The drawing under review shows one solid part. Ordinate dimensions are in mm from its lowest x, y, z. A direction names the side the tool comes from. Coordinates: 2 decimals unless noted, no trailing zeros. Order: outer loops, then holes, each group sorted by start corner. A loop starts at its lowest first (then second) coordinate and runs counter-clockwise, first axis right, second up. Notation, with made-up numbers: (39, 65) - (98, 65) arc R29 ccw to (98, 100) - close; hole circle Ø10 at (34, -11). An arc over 180 degrees is marked (long way). Write each question's results on one line, items separated by ' | '. Start each with the question number.
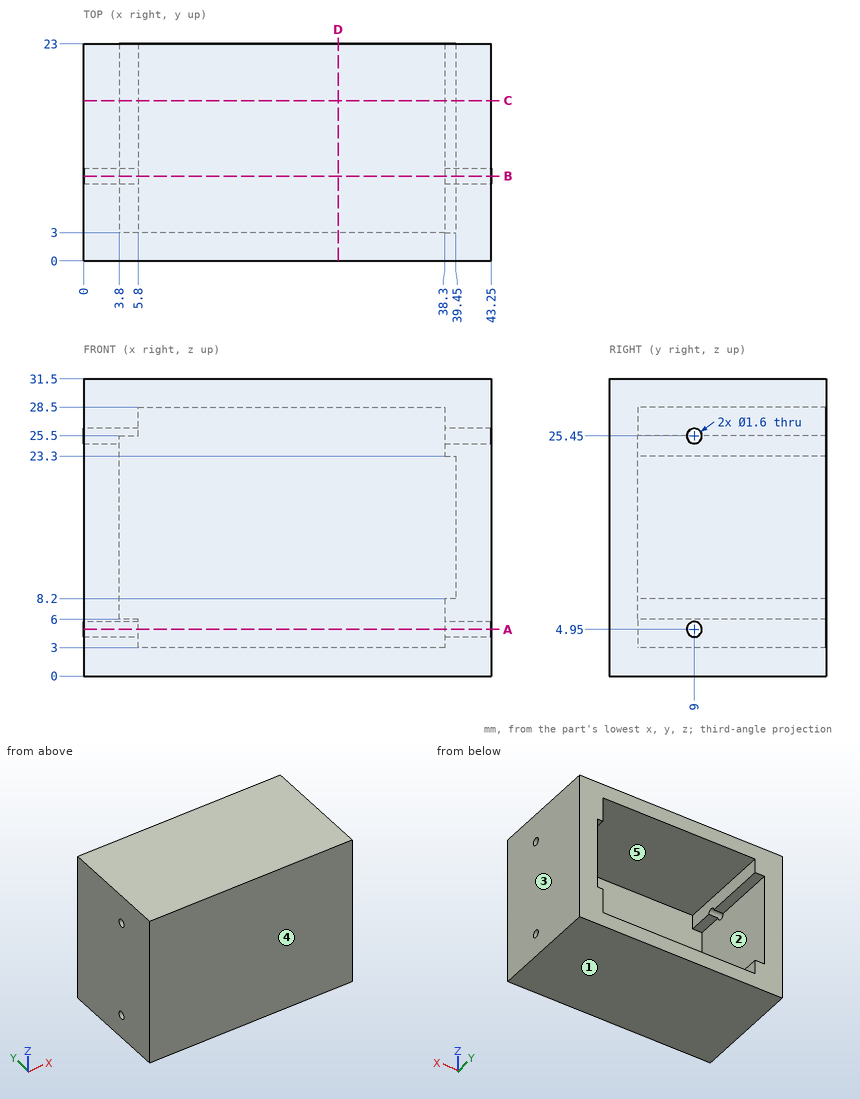
(1) Take a section at C-C (y = 17). State the section outline as (x, z) points, plus the area to 3 significant figures.
(2) To check wall thickness, follow line 1 along Z through (x, y) = (4.2, 9); line 2 along Z through (x, y) = (39.7, 9); line 3 along Y through (x, z) = (2.4, 4.95). State the ranges of each line that lie inside material, in increasing order. Write a range as [from, to].
(3) Take a section at D-D (x = 27). State the section outline as (y, z) points, plus the area to 4 significant figures.
(4) Take a section at B-B (y = 9). State how many separate pieces and enclosed holes the cut face has, plus the area to 3 significant figures.
(5) Mouldability with a two-part tool opening along X and no side actions: class the marked faces 1, 2 and 3 as +X half, -X half, draft (parallel to the pull), parting line (faces both ways), or undercut.
(6) Tool access review of the marked faces 4 and 5: name each direction out of +Z, -Z, +X, -X, +Y, -Y from which nothing blocks a thin tool from reaching the whole face with its end or side.
(7) Take a section at A-A (z = 4.95). State the section outline as (x, y) points, plus the area to 3 significant figures.
(8) Clearance check with flat-ended pins moving along their axes: pin 1 (1.3 mm diameter, centred on y = 9, z = 25.45, fed in from +X); pin 2 (5 mm diameter, centred on x = 8, z = 20, fed in from +Y). State where each tip first meets the part, or that it passes through.
Worked out:
1) outline: (0, 0) - (43.25, 0) - (43.25, 31.5) - (0, 31.5) - close; hole (3.8, 6) - (5.8, 6) - (5.8, 3) - (38.3, 3) - (38.3, 8.2) - (39.45, 8.2) - (39.45, 23.3) - (38.3, 23.3) - (38.3, 28.5) - (5.8, 28.5) - (5.8, 25.5) - (3.8, 25.5) - close | area: 477 mm^2
2) line 1: [0, 4.15], [5.75, 6], [26.25, 31.5] | line 2: [0, 4.15], [5.75, 24.65], [26.25, 31.5] | line 3: [0, 8.2], [9.8, 23]
3) outline: (0, 0) - (23, 0) - (23, 3) - (3, 3) - (3, 28.5) - (23, 28.5) - (23, 31.5) - (0, 31.5) - close | area: 214.5 mm^2
4) separate pieces: 4 | enclosed holes: 0 | area: 445 mm^2
5) face 1: draft | face 2: undercut | face 3: +X half
6) face 4: +Z, -Z, +X, -X, -Y | face 5: +Y
7) outline: (0, 0) - (43.25, 0) - (43.25, 8.2) - (38.3, 8.2) - (38.3, 3) - (5.8, 3) - (5.8, 8.2) - (0, 8.2) - close; (0, 9.8) - (5.8, 9.8) - (5.8, 23) - (0, 23) - close; (38.3, 9.8) - (43.25, 9.8) - (43.25, 23) - (38.3, 23) - close | area: 328 mm^2
8) pin 1: through | pin 2: y = 3
